Could you check a few things on this drawing? It's one solid part, dimensions in mm from its lowest x, y, z. Give positions to 0.01 mm unless a question says otherwise; leave off trailing zeros. Write each loop counter-clockwise with the first axis right and the second up, starting at its lowest first coordinate (ties: lowest second). Pieces come first, ordered by that corner, then holes. Notation, with made-up numbers: (79, 12.25) - (98, 12.25) arc R31 cw to (98, 39.25) - close; hole circle Ø1 at (-20.5, 33). An arc over 180 degrees is marked (long way). One line per item, written item: value. Start each with the question number.
1) Imagine slicing it at A-A on y = 25. Write out the boundary of the cut face in (x, z), plus the area to 3 significant figures.
2) Imagine slicing it at B-B on x = 5. Write out the boundary of the cut face in (y, z), plus the area to 3 significant figures.
3) Imagine slicing it at C-C on z = 1.6. Write out the boundary of the cut face in (x, y), plus the area to 3 significant figures.
4) Please list where these lines run through material, in increasing order: L1, parallel to Y at x = 5, z = 1.15; L2, parallel to Y at x = 4, z = 2.4; L3, parallel to Y at x = 8.75, z = 1.35. Write a range as [from, to].
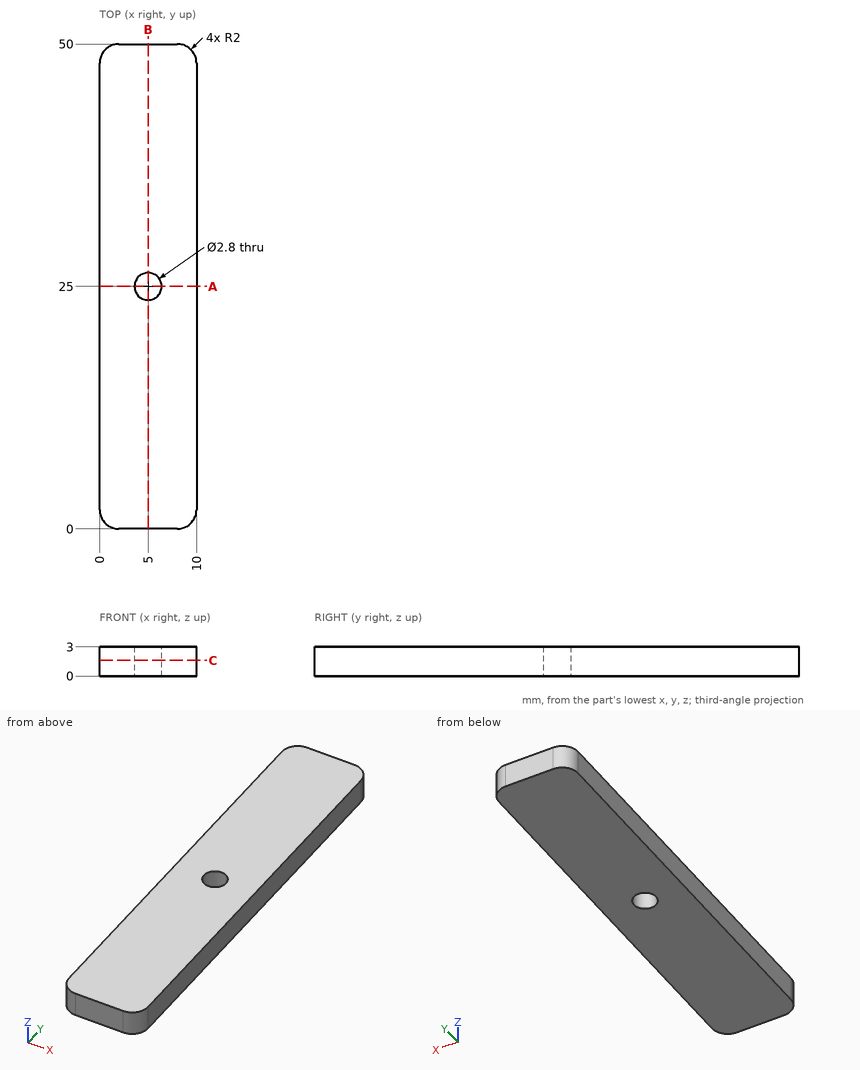
Numbers:
1. outline: (0, 0) - (3.6, 0) - (3.6, 3) - (0, 3) - close; (6.4, 0) - (10, 0) - (10, 3) - (6.4, 3) - close
1. area: 21.6 mm^2
2. outline: (0, 0) - (23.6, 0) - (23.6, 3) - (0, 3) - close; (26.4, 0) - (50, 0) - (50, 3) - (26.4, 3) - close
2. area: 142 mm^2
3. outline: (0, 2) arc R2 ccw to (2, 0) - (8, 0) arc R2 ccw to (10, 2) - (10, 48) arc R2 ccw to (8, 50) - (2, 50) arc R2 ccw to (0, 48) - close; hole circle Ø2.8 at (5, 25)
3. area: 490 mm^2
4. L1: [0, 23.6], [26.4, 50]
4. L2: [0, 24.02], [25.98, 50]
4. L3: [0.15, 49.85]
